from build123d import *

# Parameters (mm, degrees)
SKETCH1_R              = 4.5
EXTRUDE1_DEPTH         = 4
PROCESS_BENDS1_START   = -122
PROCESS_BENDS1_DEPTH   = 244
PROCESS_BENDS1_2_DEPTH = 244
PROCESS_BENDS1_START_2 = 357.035547254
PROCESS_BENDS1_3_DEPTH = 4.964452746


with BuildPart() as part:
    # Sketch1 → Extrude1 (new body)
    with BuildSketch(Plane.XY):
        with BuildLine():
            Line((-60, 0), (60, 0))
            ThreePointArc((60, 0), (61.019968244, 0.040074661), (62.033648046, 0.160051572))
            Line((62.033648046, 0.160051572), (113.56434465, 8.321712114))
            ThreePointArc((113.56434465, 8.321712114), (119.604059656, 11.704115036), (122, 18.19859552))
            Line((122, 18.19859552), (122, 405))
            ThreePointArc((122, 405), (119.071067812, 412.071067812), (112, 415))
            Line((112, 415), (-112, 415))
            ThreePointArc((-112, 415), (-119.071067812, 412.071067812), (-122, 405))
            Line((-122, 405), (-122, 18.19859552))
            ThreePointArc((-122, 18.19859552), (-119.604059656, 11.704115036), (-113.56434465, 8.321712114))
            Line((-113.56434465, 8.321712114), (-62.033648046, 0.160051572))
            ThreePointArc((-62.033648046, 0.160051572), (-61.019968244, 0.040074661), (-60, 0))
        make_face()
        with Locations((60, 13)):
            Circle(SKETCH1_R, mode=Mode.SUBTRACT)
        with Locations(Location((-60, 13, 0), (0, 0, 180))):
            Circle(SKETCH1_R, mode=Mode.SUBTRACT)
    extrude(amount=EXTRUDE1_DEPTH)

    # Process-Bends1: read off the stored shape, not the designer's step
    # Process-Bends1 outline → Process-Bends1 (cut)
    with BuildSketch(Plane.YZ.offset(PROCESS_BENDS1_START)):
        with BuildLine():
            Line((415, 4), (43.866625588, 4))
            ThreePointArc((43.866625588, 4), (41.283727655, 1.083920217), (37.542070268, 0))
            Line((37.542070268, 0), (415, 0))
            Line((415, 0), (415, 4))
        make_face()
    extrude(amount=PROCESS_BENDS1_DEPTH, mode=Mode.SUBTRACT)

    # Process-Bends1 2 outline → Process-Bends1 2 (add)
    with BuildSketch(Plane.YZ.offset(PROCESS_BENDS1_START)):
        with BuildLine():
            Line((333.473997554, 167.613261682), (329.561407151, 166.781614919))
            Line((329.561407151, 166.781614919), (332.399683469, 153.428574691))
            ThreePointArc((332.399683469, 153.428574691), (331.56796846, 150.665088271), (328.790387504, 149.881729425))
            Line((328.790387504, 149.881729425), (264.309892155, 164.768224749))
            ThreePointArc((264.309892155, 164.768224749), (261.942812278, 164.902637285), (259.666636747, 164.239192619))
            Line((259.666636747, 164.239192619), (73.570894156, 73.474234364))
            ThreePointArc((73.570894156, 73.474234364), (71.646739039, 72.08904089), (70.295337674, 70.141003872))
            Line((70.295337674, 70.141003872), (40.260993629, 5.732145215))
            ThreePointArc((40.260993629, 5.732145215), (39.153969093, 4.469825663), (37.542070268, 4))
            Line((37.542070268, 4), (43.866625588, 4))
            ThreePointArc((43.866625588, 4), (43.876459451, 4.020819967), (43.886224777, 4.041672168))
            Line((43.886224777, 4.041672168), (73.920568822, 68.450530825))
            ThreePointArc((73.920568822, 68.450530825), (74.499740836, 69.285403833), (75.324378743, 69.879058179))
            Line((75.324378743, 69.879058179), (261.420121334, 160.644016434))
            ThreePointArc((261.420121334, 160.644016434), (262.395625133, 160.928349862), (263.410087937, 160.87074449))
            Line((263.410087937, 160.87074449), (327.890583287, 145.984249165))
            ThreePointArc((327.890583287, 145.984249165), (334.371605517, 147.812086475), (336.312273872, 154.260221455))
            Line((336.312273872, 154.260221455), (333.473997554, 167.613261682))
        make_face()
    extrude(amount=PROCESS_BENDS1_2_DEPTH)

    # Process-Bends1 3 outline → Process-Bends1 3 (cut)
    with BuildSketch(Plane(origin=(0, 0, 0), x_dir=(1, 0, 0), z_dir=(0, 0.9781476007338049, 0.20791169081776298)).offset(PROCESS_BENDS1_START_2)):
        with BuildLine():
            Line((-122, -94.61736709), (-112, -94.61736709))
            ThreePointArc((-112, -94.61736709), (-119.071067812, -91.688434902), (-122, -84.61736709))
            Line((-122, -84.61736709), (-122, -94.61736709))
        make_face()
        with BuildLine():
            ThreePointArc((122, -84.61736709), (119.071067812, -91.688434902), (112, -94.61736709))
            Line((112, -94.61736709), (122, -94.61736709))
            Line((122, -94.61736709), (122, -84.61736709))
        make_face()
    extrude(amount=PROCESS_BENDS1_3_DEPTH, mode=Mode.SUBTRACT)


solid = part.part
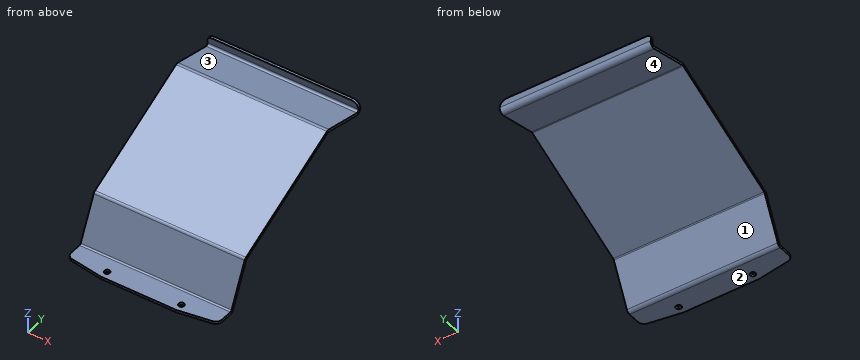
Model file for the job. Use its own axes, mm. Face numbers are marked on the shaded views. Give positions to 0.01 mm unless a question says otherwise; leave off trailing zeros. Order: outer loops, then holes, each group sorted by start corner. A loop starts at its lowest first (then second) coordinate and runs counter-clockwise, first axis right, second up. Notation, with made-up numbers: M 89,-27 L 131,-27 A16 ccw 131,2 Z; hole C -30.5,5.5 d2. An arc over 180 degrees is marked long. Put each result on its own line as item: value. Start each with the question number.
(1) Band-saw the part on C-C on x = -76. Give the cut face in (y, z).
(2) Band-saw the part on A-A on x = 36. Give the cut face in (y, z).
(3) Band-saw the part on D-D on y = 304.5. Give the cut face in (x, z).
(4) Drill centre lines: L1, parallel to Z at x = -72, y = 31.5; L2, parallel to Y at x = 60, z = 2.5; L3, parallel to Y at x = -60, z = 2. Where is each one in solid material? Low to high. Write a range as [from, to].
(5) Pin check, flat tips, straight feed: pin 1 Ø19 at (x, y) = (-2.5, 23) entering from +Z; pin 2 Ø1.5 at (x, z) = (-93, 39) entering from -Y; pin 3 Ø1 at (x, z) = (26.5, 87.5) entering from -Y. Stop position of each tip, or through.
(6) Band-saw the part on B-B on y = 13. Give the cut face in (x, z), then the cut area to 3 significant figures.
(7) Pull direction Y, two halves, no side cores. Call the marked faces 1, 2, 3 and 4: released by +Y, released by -Y, zero draft, split by the parting line, or undercut.
Results below:
1. outline: M 2.37,0 L 37.54,0 A7 ccw 43.87,4 A7 ccw 43.89,4.04 L 73.92,68.45 A3 cw 75.32,69.88 L 261.42,160.64 A3 cw 263.41,160.87 L 327.89,145.98 A7 ccw 336.31,154.26 L 333.47,167.61 L 329.56,166.78 L 332.4,153.43 A3 cw 328.79,149.88 L 264.31,164.77 A7 ccw 259.67,164.24 L 73.57,73.47 A7 ccw 70.3,70.14 L 40.26,5.73 A3 cw 37.54,4 L 2.37,4 Z
2. outline: M 0,0 L 37.54,0 A7 ccw 43.87,4 A7 ccw 43.89,4.04 L 73.92,68.45 A3 cw 75.32,69.88 L 261.42,160.64 A3 cw 263.41,160.87 L 327.89,145.98 A7 ccw 336.31,154.26 L 333.47,167.61 L 329.56,166.78 L 332.4,153.43 A3 cw 328.79,149.88 L 264.31,164.77 A7 ccw 259.67,164.24 L 73.57,73.47 A7 ccw 70.3,70.14 L 40.26,5.73 A3 cw 37.54,4 L 0,4 Z
3. outline: M -122,151.38 L 122,151.38 L 122,155.49 L -122,155.49 Z
4. L1: z = [0, 4]
4. L2: y = [0, 8.5], [17.5, 42.9]
4. L3: y = [0, 8.5], [17.5, 42.44]
5. pin 1: stops at z = 4
5. pin 2: stops at y = 55.42
5. pin 3: stops at y = 101.3
6. outline: M -120.54,0 L -64.5,0 L -64.5,4 L -120.54,4 Z; M -55.5,0 L 55.5,0 L 55.5,4 L -55.5,4 Z; M 64.5,0 L 120.54,0 L 120.54,4 L 64.5,4 Z
6. area: 892 mm2
7. face 1: released by +Y
7. face 2: zero draft
7. face 3: undercut
7. face 4: undercut
